Work out the finished part from the listing and answer in its coordinate system (mm). Face numbers are marked on the shaded views. A direction names the side the tool comes from. Give positions to 0.01 mm unless a question says otherwise; leave off trailing zeros. Loops run counter-clockwise (first coordinate to the right, second up) from the corner with the lowest first, then second, coordinate; pieces in that order, holes last. Notation, with made-up numbers: (-35, 30) - (6, 30) arc R30 cw to (6, 65) - close; hole circle Ø5 at (33, 56.25). An arc over 180 degrees is marked (long way). One line per item, written item: value.
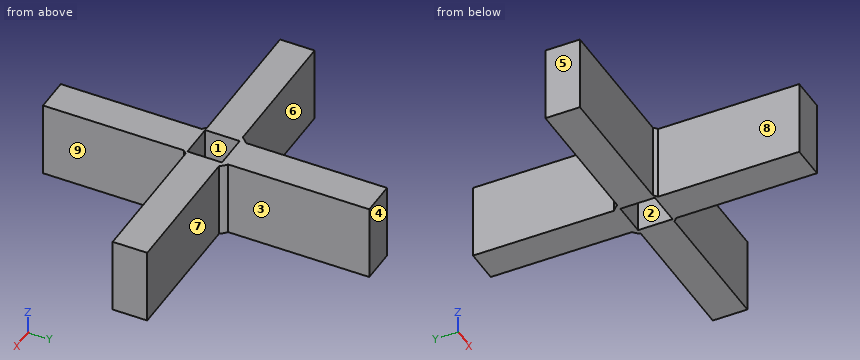
from build123d import *

# Parameters (mm, degrees)
F1_DEPTH = 2


# Not quite as in the source:
# - the program builds the solid bodies; features that only make, move or delete a surface that nothing else refers to are left out


with BuildPart() as f1:
    # F0 (on Top) → F1 (new body)
    with BuildSketch(Plane.XY):
        with BuildLine():
            ThreePointArc((0.5437049493, -0.4874087926), (0.6819795338, -0.2609335518), (0.7301934011, 0))
            ThreePointArc((0.7301934011, 0), (0.697527915, 0.2159565019), (0.6024540634, 0.4125912074))
            Line((0.6024540634, 0.4125912074), (0.45, 0.4125912074))
            Line((0.45, 0.4125912074), (0.45, -0.4874087926))
            Line((0.45, -0.4874087926), (0.5437049493, -0.4874087926))
        make_face()
        with BuildLine():
            ThreePointArc((0.6024540634, 0.4125912074), (0.697527915, 0.2159565019), (0.7301934011, 0))
            ThreePointArc((0.7301934011, 0), (0.6819795338, -0.2609335518), (0.5437049493, -0.4874087926))
            Line((0.5437049493, -0.4874087926), (4.2458724273, -0.4874087926))
            Line((4.2458724273, -0.4874087926), (4.2458724273, 0.4125912074))
            Line((4.2458724273, 0.4125912074), (0.6024540634, 0.4125912074))
        make_face()
        with BuildLine():
            Line((0.45, 0.4125912074), (0.6024540634, 0.4125912074))
            ThreePointArc((0.6024540634, 0.4125912074), (0.5324594789, 0.4996691968), (0.45, 0.5750499134))
            Line((0.45, 0.5750499134), (0.45, 0.4125912074))
        make_face()
        with BuildLine():
            ThreePointArc((0.45, -0.5750499134), (0.4987811374, -0.5332914587), (0.5437049493, -0.4874087926))
            Line((0.5437049493, -0.4874087926), (0.45, -0.4874087926))
            Line((0.45, -0.4874087926), (0.45, -0.5750499134))
        make_face()
        with BuildLine():
            Line((0.45, 0.4125912074), (0.45, 0.5750499134))
            ThreePointArc((0.45, 0.5750499134), (0, 0.7301934011), (-0.45, 0.5750499134))
            Line((-0.45, 0.5750499134), (-0.45, 0.4125912074))
            Line((-0.45, 0.4125912074), (0.45, 0.4125912074))
        make_face()
        with BuildLine():
            ThreePointArc((-0.45, 0.5750499134), (0, 0.7301934011), (0.45, 0.5750499134))
            Line((0.45, 0.5750499134), (0.45, 4.25))
            Line((0.45, 4.25), (-0.45, 4.25))
            Line((-0.45, 4.25), (-0.45, 0.5750499134))
        make_face()
        with BuildLine():
            Line((0.45, -4.25), (0.45, -0.5750499134))
            ThreePointArc((0.45, -0.5750499134), (0, -0.7301934011), (-0.45, -0.5750499134))
            Line((-0.45, -0.5750499134), (-0.45, -4.25))
            Line((-0.45, -4.25), (0.45, -4.25))
        make_face()
        with BuildLine():
            ThreePointArc((-0.45, -0.5750499134), (0, -0.7301934011), (0.45, -0.5750499134))
            Line((0.45, -0.5750499134), (0.45, -0.4874087926))
            Line((0.45, -0.4874087926), (-0.45, -0.4874087926))
            Line((-0.45, -0.4874087926), (-0.45, -0.5750499134))
        make_face()
        with BuildLine():
            Line((-0.45, 0.4125912074), (-0.45, 0.5750499134))
            ThreePointArc((-0.45, 0.5750499134), (-0.5324594789, 0.4996691968), (-0.6024540634, 0.4125912074))
            Line((-0.6024540634, 0.4125912074), (-0.45, 0.4125912074))
        make_face()
        with BuildLine():
            Line((-0.45, -0.4874087926), (-0.45, 0.4125912074))
            Line((-0.45, 0.4125912074), (-0.6024540634, 0.4125912074))
            ThreePointArc((-0.6024540634, 0.4125912074), (-0.7286426563, -0.0475634562), (-0.5437049493, -0.4874087926))
            Line((-0.5437049493, -0.4874087926), (-0.45, -0.4874087926))
        make_face()
        with BuildLine():
            ThreePointArc((-0.5437049493, -0.4874087926), (-0.4987811374, -0.5332914587), (-0.45, -0.5750499134))
            Line((-0.45, -0.5750499134), (-0.45, -0.4874087926))
            Line((-0.45, -0.4874087926), (-0.5437049493, -0.4874087926))
        make_face()
        with BuildLine():
            ThreePointArc((-0.5437049493, -0.4874087926), (-0.7286426563, -0.0475634562), (-0.6024540634, 0.4125912074))
            Line((-0.6024540634, 0.4125912074), (-4.2537945996, 0.4125912074))
            Line((-4.2537945996, 0.4125912074), (-4.2537945996, -0.4874087926))
            Line((-4.2537945996, -0.4874087926), (-0.5437049493, -0.4874087926))
        make_face()
    extrude(amount=F1_DEPTH)


solid = f1.part
1. Section A-A (z = 1.5) is taken. Write down the section's boundary in (x, y).
Output:
outline: (-4.25, -0.49) - (-0.54, -0.49) arc R0.73 ccw to (-0.45, -0.58) - (-0.45, -4.25) - (0.45, -4.25) - (0.45, -0.58) arc R0.73 ccw to (0.54, -0.49) - (4.25, -0.49) - (4.25, 0.41) - (0.6, 0.41) arc R0.73 ccw to (0.45, 0.58) - (0.45, 4.25) - (-0.45, 4.25) - (-0.45, 0.58) arc R0.73 ccw to (-0.6, 0.41) - (-4.25, 0.41) - close; hole (-0.45, -0.49) - (0.45, -0.49) - (0.45, 0.41) - (-0.45, 0.41) - close
2. Find the intervals of material crossed by line 1 along Y through (x, z) = (2, 1.65); line 2 along X through (y, z) = (1.5, 1.5), in increasing order.
Output:
line 1: y = -0.49 to 0.41
line 2: x = -0.45 to 0.45
3. The mould has two halves that part along Y. Classify the marked faces 1, 2, 3 and 4: released by +Y, released by -Y, zero draft, split by the parting line, or undercut.
Output:
face 1: undercut
face 2: undercut
face 3: zero draft
face 4: released by +Y
4. Section B-B (x = -2.5) is taken. Write down the section's boundary in (y, z).
Output:
outline: (-0.49, 0) - (0.41, 0) - (0.41, 2) - (-0.49, 2) - close
5. Flat-ended cylindrical pins translate along their axes: pin 1 Ø0.6 at (x, z) = (1.5, 1) entering from -Y; pin 2 Ø1 at (x, z) = (-3, 1.5) entering from +Y; pin 3 Ø0.6 at (y, z) = (2.5, 1) entering from +X. Find the tip coordinate at first contact, or state that the pin passes through.
Output:
pin 1: stops at y = -0.49
pin 2: stops at y = 0.41
pin 3: stops at x = 0.45
6. For the marked faces 5, 6, 7, 8 and 9, determine the directions among +Z, -Z, +X, -X, +Y, -Y from which every point of the face is accessible in a straight line to the end or side of a thin tool.
Output:
face 5: +Z, -Z, -X, +Y, -Y
face 6: +Z, -Z, -X, +Y
face 7: +Z, -Z, +X, +Y
face 8: +Z, -Z, -X, -Y
face 9: +Z, -Z, +X, -Y
7. Section C-C (y = -0.75) is taken. Write down the section's boundary in (x, z).
Output:
outline: (-0.45, 0) - (0.45, 0) - (0.45, 2) - (-0.45, 2) - close
